The figure shows three views and two pictorial views of one solid part (mm, origin at its lowest corner). Answer the questions. Coordinates: 2 decimals unless noted, no trailing zeros. Order: outer loops, then holes, each group sorted by start corner. A loop starts at its lowest first (then second) coordinate and runs counter-clockwise, first axis right, second up.
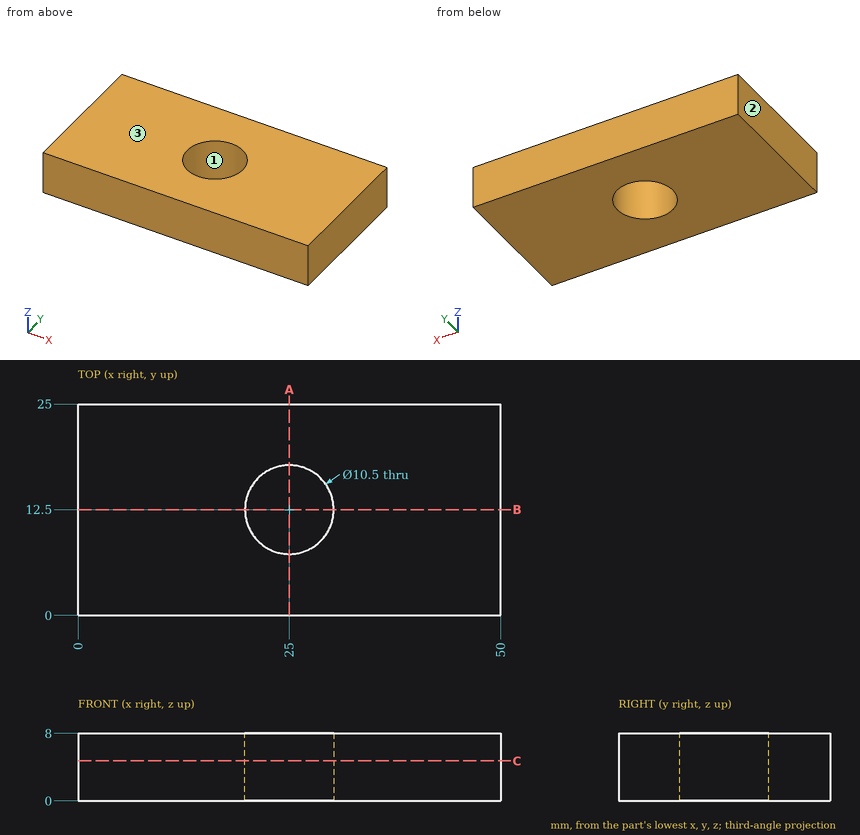
Q1. The part is cut by section B-B, the plane y = 12.5. Determine the outline of the cut face in (x, z).
Q2. Determine the mould class of the marked faces 1, 2 and 3 for opening direction X: +X half, -X half, draft (parallel to the pull), parting line (faces both ways), or undercut.
Q3. This flat-tipped pin is pushed along its axis until it touches: P1, Ø3, axis at x = 41, y = 12.5, coming from the -Z side. Where does it stop, or does it pass through?
Q4. Straight lines are drawn through the part: L1, parallel to Y at x = 25, z = 3.25; L2, parallel to X at y = 8, z = 3; L3, parallel to X at y = 15, z = 5. For each, find the intervals that lie inside material, in ascending order.
Q5. The part is cut by section A-A, the plane x = 25. Determine the outline of the cut face in (y, z), then the cut area to 3 significant figures.
Q6. The part is cut by section C-C, the plane z = 4.75. Determine the outline of the cut face in (x, y).
Computed values:
1. outline: (0, 0) - (19.75, 0) - (19.75, 8) - (0, 8) - close; (30.25, 0) - (50, 0) - (50, 8) - (30.25, 8) - close
2. face 1: undercut
2. face 2: -X half
2. face 3: draft
3. P1: stops at z = 0
4. L1: y = 0 to 7.25, 17.75 to 25
4. L2: x = 0 to 22.3, 27.7 to 50
4. L3: x = 0 to 20.38, 29.62 to 50
5. outline: (0, 0) - (7.25, 0) - (7.25, 8) - (0, 8) - close; (17.75, 0) - (25, 0) - (25, 8) - (17.75, 8) - close
5. area: 116 mm2
6. outline: (0, 0) - (50, 0) - (50, 25) - (0, 25) - close; hole circle Ø10.5 at (25, 12.5)
